Input: dimensioned drawing with shaded views. Units: mm. Origin: part minimum x, y, z. A direction names the side the tool comes from. Give positions to 0.01 mm unless a question says otherwise; leave off trailing zeros. Write each loop counter-clockwise with the first axis right and the second up, starting at its lowest first coordinate (ties: lowest second). Pieces come first, ordered by that corner, then holes. Notation, with made-up numbers: (59, 17) -> (114, 17) arc R23 ccw to (114, 45) -> close; hole circle Ø3 at (42.5, 50). An arc over 180 degrees is marked (long way). Answer as a JSON object with one key per item and string values. Group by question number.
(1) Draft query along Y for the marked faces 3, 4 and 5. Return one class per face: +Y half, -Y half, draft (parallel to the pull), parting line (faces both ways), or undercut.
(2) Section query D-D on x = 3.75. Output: boundary loops of the cut face in (y, z), plus the area to 3 significant figures.
(3) Set-up query: the marked faces 1 and 2. Return all of +Z, -Z, +X, -X, +Y, -Y with unobstructed straight access to the full face (end or side cutting, diameter ignored); none if empty.
(4) Section query A-A on z = 5.5. Output: boundary loops of the cut face in (x, y), plus the area to 3 significant figures.
(5) Section query C-C on x = 9. Output: boundary loops of the cut face in (y, z).
(6) Section query B-B on y = 10.25. Output: boundary loops of the cut face in (x, z).
(7) Material intervals for probe 1 along Y at (x, z) = (9, 6.25); probe 2 along Z at (x, y) = (1.5, 4.75); probe 3 along Y at (x, z) = (1.25, 6.5), sorted ascending.
(8) Contact query for flat-ended pins moving along their axis: pin 1 Ø2.5 at (y, z) = (11, 8.5) entering from -X; pin 2 Ø5 at (x, y) = (10, 17.5) entering from -Z; pin 3 Ø3.5 at (x, y) = (9, 10.25) entering from -Z. Output: stop coordinate, or through.
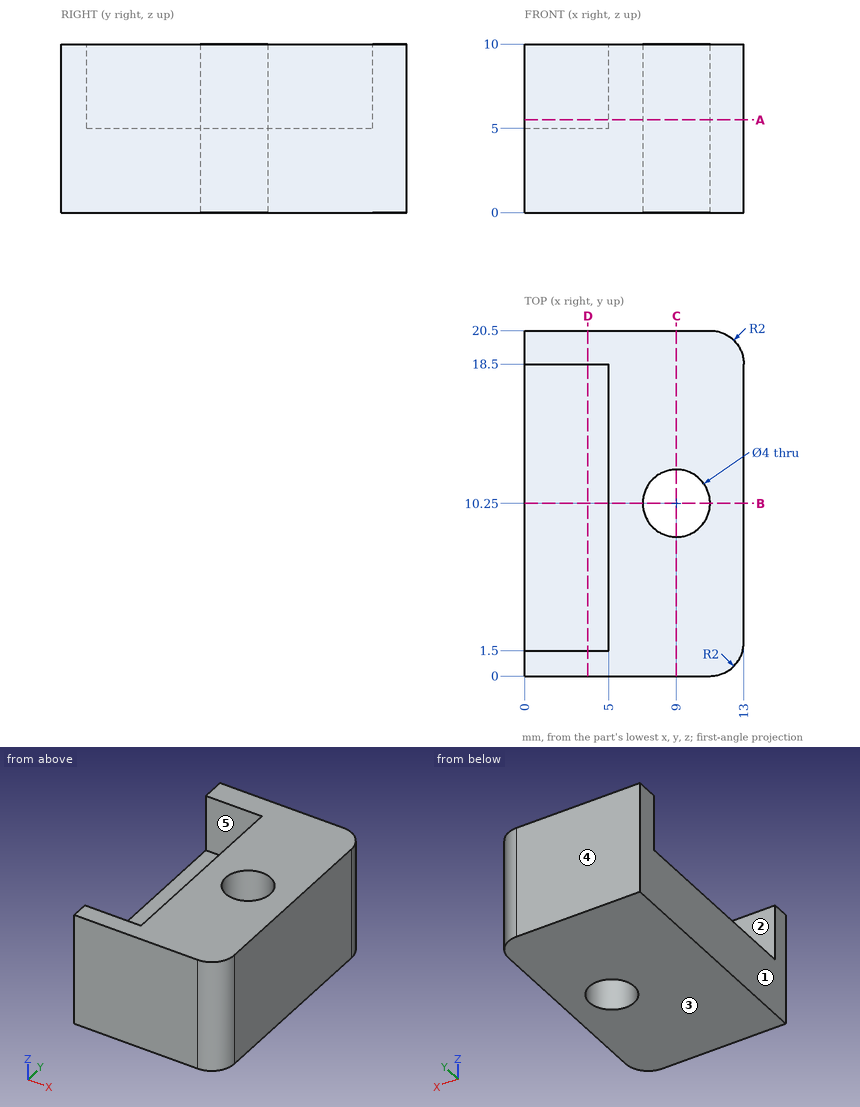
Answer list:
{
 "1": {"face 3": "draft", "face 4": "+Y half", "face 5": "undercut"},
 "2": {"outline": "(0, 0) -> (20.5, 0) -> (20.5, 10) -> (18.5, 10) -> (18.5, 5) -> (1.5, 5) -> (1.5, 10) -> (0, 10) -> close", "area": "120 mm2"},
 "3": {"face 1": "+Z, -Z, -X, +Y, -Y", "face 2": "+Z, -X"},
 "4": {"outline": "(0, 0) -> (11, 0) arc R2 ccw to (13, 2) -> (13, 18.5) arc R2 ccw to (11, 20.5) -> (0, 20.5) -> (0, 18.5) -> (5, 18.5) -> (5, 1.5) -> (0, 1.5) -> close; hole circle Ø4 at (9, 10.25)", "area": "167 mm2"},
 "5": {"outline": "(0, 0) -> (8.25, 0) -> (8.25, 10) -> (0, 10) -> close; (12.25, 0) -> (20.5, 0) -> (20.5, 10) -> (12.25, 10) -> close"},
 "6": {"outline": "(0, 0) -> (7, 0) -> (7, 10) -> (5, 10) -> (5, 5) -> (0, 5) -> close; (11, 0) -> (13, 0) -> (13, 10) -> (11, 10) -> close"},
 "7": {"probe 1": "0 to 8.25, 12.25 to 20.5", "probe 2": "0 to 5", "probe 3": "0 to 1.5, 18.5 to 20.5"},
 "8": {"pin 1": "x = 5", "pin 2": "z = 0", "pin 3": "through"}
}
